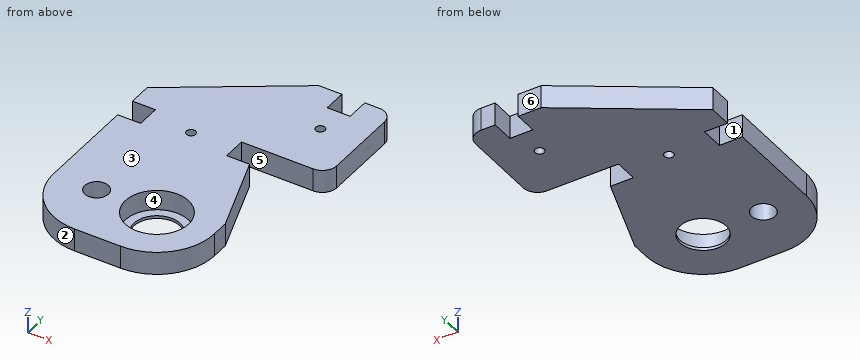
from build123d import *

# Parameters (mm, degrees)
CYLINDER_R     = 11
CYLINDER_DEPTH = 7
SKETCH_R       = 4.1
SKETCH_R_2     = 8
SKETCH_R_3     = 1.6
PAD_DEPTH      = 8


with BuildPart() as cylinder:
    # Cylinder → Cylinder (new body)
    with BuildSketch(Plane.XY.offset(1)):
        Circle(CYLINDER_R)
    extrude(amount=CYLINDER_DEPTH)


with BuildPart() as cut:
    # Sketch → Pad (new body)
    with BuildSketch(Plane.XY):
        with BuildLine():
            Line((1e-06, -20), (-16, -20))
            ThreePointArc((-36, 0), (-30.142135, -14.142136), (-16, -20))
            Line((-36, 0), (-36, 34.95))
            Line((-28, 34.95), (-36, 34.95))
            Line((-28, 39), (-28, 34.95))
            Line((-28, 39), (-28, 43.05))
            Line((-28, 43.05), (-36, 43.05))
            Line((-36, 51.05), (-36, 43.05))
            Line((-36, 51.05), (6, 79.05))
            Line((6, 79.05), (14, 79.05))
            Line((14, 79.05), (14, 71.05))
            Line((14, 71.05), (18, 71.05))
            Line((18, 71.05), (22, 71.05))
            Line((22, 71.05), (22, 79.05))
            Line((22, 79.05), (27, 79.05))
            ThreePointArc((32, 74.05), (30.535534, 77.585534), (27, 79.05))
            Line((32, 48.05), (32, 74.05))
            ThreePointArc((27, 43.05), (30.535534, 44.514466), (32, 48.05))
            Line((2, 43.05), (27, 43.05))
            Line((2, 39), (2, 43.05))
            Line((2, 34.95), (2, 39))
            Line((2, 34.95), (10, 34.95))
            Line((10, 34.95), (20, 6))
            Line((20, 0), (20, 6))
            ThreePointArc((1e-06, -20), (14.142136, -14.142136), (20, 0))
        make_face()
        with Locations((-21, 0)):
            Circle(SKETCH_R, mode=Mode.SUBTRACT)
        with Locations((0, 0)):
            Circle(SKETCH_R_2, mode=Mode.SUBTRACT)
        with Locations((-13, 39)):
            Circle(SKETCH_R_3, mode=Mode.SUBTRACT)
        with Locations((18, 61.05)):
            Circle(SKETCH_R_3, mode=Mode.SUBTRACT)
    extrude(amount=PAD_DEPTH)

    # Cut: cut Cylinder
    add(cylinder.part, mode=Mode.SUBTRACT)


solid = cut.part
CAD build for the part. Positions are in the model's coordinates, mm. Face numbers are marked on the shaded views. A direction names the side the tool comes from. Round coordinates to 2 decimals unless told otherwise and drop trailing zeros. Loops run counter-clockwise (first coordinate to the right, second up) from the corner with the lowest first, then second, coordinate; pieces in that order, holes last. Notation, with made-up numbers: M 69.25,-29.5 L 112.25,-29.5 A19 cw 112.25,-7.5 Z; hole C 86.25,14.25 d10. An arc over 180 degrees is marked long. One line per question, with ' | ' between items. Start each with the question number.
Item 1: Cut at A-A, the plane y = 39. Write the cut outline in (x, z), plus the area to 3 significant figures.
Item 2: Cut at C-C, the plane x = 18. Write the cut outline in (y, z), plus the area to 3 significant figures.
Item 3: Which spindle directions (+Z, -Z, +X, -X, +Y, -Y) get a long thin tool onto all of the face, cutting with end or side? Do the marked faces 4, 5 and 6. Say none if no direction does.
Item 4: Two-plate mould, pull along Y, no slides. Class the marked faces 1, 2 and 3: pulls with the +Y half, pulls with the -Y half, needs draft (parallel to the pull), parting line crosses it, or undercut.
Item 5: Pin check, flat tips, straight feed: pin 1 Ø4 at (x, y) = (-1, -6) entering from +Z; pin 2 Ø6.5 at (x, y) = (0.5, 3.5) entering from +Z; pin 3 Ø4 at (y, z) = (77, 5.5) entering from +X; pin 4 Ø2.5 at (x, z) = (18.5, 4) entering from -Y. Stop position of each tip, or through.
Item 6: Cut at B-B, the plane z = 2.5. Write the cut outline in (x, y).
Item 7: Wall check: line 1 (Y direction, x = -30, z = 3.75); line 2 (Y direction, x = 4.5, z = 4); line 3 (Y direction, x = -21, z = 4.5). Give the ranges that are in metal, low to high.
Item 8: Cut at D-D, the plane x = -30. Write the cut outline in (y, z), plus the area to 3 significant figures.
Responses:
1) outline: M -28,0 L -14.6,0 L -14.6,8 L -28,8 Z; M -11.4,0 L 2,0 L 2,8 L -11.4,8 Z | area: 214 mm²
2) outline: M -8.72,0 L 11.79,0 L 11.79,8 L -8.72,8 Z; M 43.05,0 L 59.45,0 L 59.45,8 L 43.05,8 Z; M 62.65,0 L 71.05,0 L 71.05,8 L 62.65,8 Z | area: 362 mm²
3) face 4: +Z | face 5: +Z, -Z, +X | face 6: +Z, -Z, +X, -X, +Y
4) face 1: undercut | face 2: pulls with the -Y half | face 3: needs draft
5) pin 1: stops at z = 1 | pin 2: passes through | pin 3: stops at x = 31.91 | pin 4: stops at y = -10.12
6) outline: M -36,0 A20 ccw -16,-20 L 0,-20 A20 ccw 20,0 L 20,6 L 10,34.95 L 2,34.95 L 2,43.05 L 27,43.05 A5 ccw 32,48.05 L 32,74.05 A5 ccw 27,79.05 L 22,79.05 L 22,71.05 L 14,71.05 L 14,79.05 L 6,79.05 L -36,51.05 L -36,43.05 L -28,43.05 L -28,34.95 L -36,34.95 Z; hole C -21,0 d8.2; hole C -13,39 d3.2; hole C 0,0 d22; hole C 18,61.05 d3.2
7) line 1: y = -14.28 to 34.95, 43.05 to 55.05 | line 2: y = -19.49 to -10.04, 10.04 to 34.95, 43.05 to 78.05 | line 3: y = -19.36 to -4.1, 4.1 to 61.05
8) outline: M -14.28,0 L 34.95,0 L 34.95,8 L -14.28,8 Z; M 43.05,0 L 55.05,0 L 55.05,8 L 43.05,8 Z | area: 490 mm²
